Autodesk Fusion 360 part; units mm, degrees
sketch "Sketch1" plane through (0, 0, 0) normal (0, 0, 1) x (1, 0, 0)
  line L0 (60, -60) -> (-60, -60)
  line L1 (-60, -60) -> (-60, 60)
  line L2 (-60, 60) -> (60, 60)
  line L3 (60, 60) -> (60, -60)
  line L4 (60, -60) -> (-60, 60) construction
  line L5 (-60, -60) -> (60, 60) construction
  dimension "d4" = 120
  dimension "d5" = 120
extrude "Extrude1" add sketch "Sketch1" along normal blind 6
sketch "Sketch6" plane through (0, 0, 6) normal (0, 0, 1) x (-1, 0, 0)
  line L0 (-60, -60) -> (60, -60)
  line L1 (60, -60) -> (60, 60)
  line L2 (60, 60) -> (-60, 60)
  line L3 (-60, 60) -> (-60, -60)
sketch "Sketch7" plane through (0, 0, 6) normal (0, 0, 1) x (-1, 0, 0)
  line L0 (-60, -60) -> (60, -60)
  line L1 (60, -60) -> (60, 60)
  line L2 (60, 60) -> (-60, 60)
  line L3 (-60, 60) -> (-60, -60)
  line L4 (50, 60) -> (40, 60)
  line L5 (40, 60) -> (40, 70)
  line L6 (40, 70) -> (50, 70)
  line L7 (50, 70) -> (50, 60)
  circle A0 centre (45, 65) radius 1.625
  line L8 (0, -80) -> (0, 80) construction
  line L9 (75, 0) -> (-75, 0) construction
  circle A1 centre (-45, 65) radius 1.625
  line L10 (-50, 60) -> (-40, 60)
  line L11 (-40, 70) -> (-50, 70)
  line L12 (-40, 60) -> (-40, 70)
  line L13 (-50, 70) -> (-50, 60)
  line L14 (40, -70) -> (50, -70)
  line L15 (0, 80) -> (0, -80) construction
  line L16 (-40, -70) -> (-50, -70)
  line L17 (50, -60) -> (40, -60)
  circle A2 centre (-45, -65) radius 1.625
  line L18 (40, -60) -> (40, -70)
  circle A3 centre (45, -65) radius 1.625
  line L19 (50, -70) -> (50, -60)
  line L20 (-40, -60) -> (-40, -70)
  line L21 (-50, -70) -> (-50, -60)
  dimension "d78" = 10
  dimension "d79" = 10
  dimension "d80" = 10
  dimension "d81" = 3.25
  dimension "d83" = 5
  dimension "d84" = 5
extrude "Extrude7" add sketch "Sketch7" against normal up to surface (6 mm away) contours L0 L16 L20 L21 | L2 L10 L11 L12 L13 | L0 L14 L17 L18 L19 | L2 L4 L5 L6 L7
fillet "Fillet1" radius 3.5 2 edges at (-50, -70, 3) (-40, -70, 3)
fillet "Fillet2" radius 3.5 2 edges at (40, -70, 3) (50, -70, 3)
fillet "Fillet3" radius 3.5 2 edges at (-40, 70, 3) (-50, 70, 3)
fillet "Fillet4" radius 3.5 2 edges at (40, 70, 3) (50, 70, 3)
fillet "Fillet5" radius 2.5 8 edges at (50, 60, 3) (40, 60, 3) (-40, 60, 3) (-50, 60, 3) (-50, -60, 3) (50, -60, 3) (-40, -60, 3) (40, -60, 3)
fillet "Fillet6" radius 3 4 edges at (-60, 60, 3) (-60, -60, 3) (60, -60, 3) (60, 60, 3)
sketch "Sketch8" plane through (0, 0, 6) normal (0, 0, 1) x (-1, 0, 0)
  circle A0 centre (45, -65) radius 1.625
  circle A1 centre (45, 65) radius 1.625
  circle A2 centre (-45, -65) radius 1.625
  circle A3 centre (-45, 65) radius 1.625
  arc A4 (-60, -57) -> (-57, -60) centre (-57, -57) ccw
  line L0 (-57, -60) -> (-52.5, -60)
  arc A5 (-50, -62.5) -> (-52.5, -60) centre (-52.5, -62.5) ccw
  line L1 (-50, -62.5) -> (-50, -66.5)
  arc A6 (-50, -66.5) -> (-46.5, -70) centre (-46.5, -66.5) ccw
  line L2 (-46.5, -70) -> (-43.5, -70)
  arc A7 (-43.5, -70) -> (-40, -66.5) centre (-43.5, -66.5) ccw
  line L3 (-40, -66.5) -> (-40, -62.5)
  arc A8 (-37.5, -60) -> (-40, -62.5) centre (-37.5, -62.5) ccw
  line L4 (-37.5, -60) -> (37.5, -60)
  arc A9 (40, -62.5) -> (37.5, -60) centre (37.5, -62.5) ccw
  line L5 (40, -62.5) -> (40, -66.5)
  arc A10 (40, -66.5) -> (43.5, -70) centre (43.5, -66.5) ccw
  line L6 (43.5, -70) -> (46.5, -70)
  arc A11 (46.5, -70) -> (50, -66.5) centre (46.5, -66.5) ccw
  line L7 (50, -66.5) -> (50, -62.5)
  arc A12 (52.5, -60) -> (50, -62.5) centre (52.5, -62.5) ccw
  line L8 (52.5, -60) -> (57, -60)
  arc A13 (57, -60) -> (60, -57) centre (57, -57) ccw
  line L9 (60, -57) -> (60, 57)
  arc A14 (60, 57) -> (57, 60) centre (57, 57) ccw
  line L10 (57, 60) -> (52.5, 60)
  arc A15 (50, 62.5) -> (52.5, 60) centre (52.5, 62.5) ccw
  line L11 (50, 62.5) -> (50, 66.5)
  arc A16 (50, 66.5) -> (46.5, 70) centre (46.5, 66.5) ccw
  line L12 (46.5, 70) -> (43.5, 70)
  arc A17 (43.5, 70) -> (40, 66.5) centre (43.5, 66.5) ccw
  line L13 (40, 66.5) -> (40, 62.5)
  arc A18 (37.5, 60) -> (40, 62.5) centre (37.5, 62.5) ccw
  line L14 (37.5, 60) -> (-37.5, 60)
  arc A19 (-40, 62.5) -> (-37.5, 60) centre (-37.5, 62.5) ccw
  line L15 (-40, 62.5) -> (-40, 66.5)
  arc A20 (-40, 66.5) -> (-43.5, 70) centre (-43.5, 66.5) ccw
  line L16 (-43.5, 70) -> (-46.5, 70)
  arc A21 (-46.5, 70) -> (-50, 66.5) centre (-46.5, 66.5) ccw
  line L17 (-50, 66.5) -> (-50, 62.5)
  arc A22 (-52.5, 60) -> (-50, 62.5) centre (-52.5, 62.5) ccw
  line L18 (-52.5, 60) -> (-57, 60)
  arc A23 (-57, 60) -> (-60, 57) centre (-57, 57) ccw
  line L19 (-60, 57) -> (-60, -57)
  circle A24 centre (45, 65) radius 2.875
  dimension "d98" = 5.75
extrude "Extrude8" cut sketch "Sketch8" against normal blind 3.5 contours A24
sketch "Sketch9" plane through (0, 0, 6) normal (0, 0, 1) x (-1, 0, 0)
  circle A0 centre (45, 65) radius 2.875
  circle A1 centre (45, -65) radius 1.625
  circle A2 centre (-45, -65) radius 1.625
  circle A3 centre (-45, 65) radius 1.625
  arc A4 (-60, -57) -> (-57, -60) centre (-57, -57) ccw
  line L0 (-57, -60) -> (-52.5, -60)
  arc A5 (-50, -62.5) -> (-52.5, -60) centre (-52.5, -62.5) ccw
  line L1 (-50, -62.5) -> (-50, -66.5)
  arc A6 (-50, -66.5) -> (-46.5, -70) centre (-46.5, -66.5) ccw
  line L2 (-46.5, -70) -> (-43.5, -70)
  arc A7 (-43.5, -70) -> (-40, -66.5) centre (-43.5, -66.5) ccw
  line L3 (-40, -66.5) -> (-40, -62.5)
  arc A8 (-37.5, -60) -> (-40, -62.5) centre (-37.5, -62.5) ccw
  line L4 (-37.5, -60) -> (37.5, -60)
  arc A9 (40, -62.5) -> (37.5, -60) centre (37.5, -62.5) ccw
  line L5 (40, -62.5) -> (40, -66.5)
  arc A10 (40, -66.5) -> (43.5, -70) centre (43.5, -66.5) ccw
  line L6 (43.5, -70) -> (46.5, -70)
  arc A11 (46.5, -70) -> (50, -66.5) centre (46.5, -66.5) ccw
  line L7 (50, -66.5) -> (50, -62.5)
  arc A12 (52.5, -60) -> (50, -62.5) centre (52.5, -62.5) ccw
  line L8 (52.5, -60) -> (57, -60)
  arc A13 (57, -60) -> (60, -57) centre (57, -57) ccw
  line L9 (60, -57) -> (60, 57)
  arc A14 (60, 57) -> (57, 60) centre (57, 57) ccw
  line L10 (57, 60) -> (52.5, 60)
  arc A15 (50, 62.5) -> (52.5, 60) centre (52.5, 62.5) ccw
  line L11 (50, 62.5) -> (50, 66.5)
  arc A16 (50, 66.5) -> (46.5, 70) centre (46.5, 66.5) ccw
  line L12 (46.5, 70) -> (43.5, 70)
  arc A17 (43.5, 70) -> (40, 66.5) centre (43.5, 66.5) ccw
  line L13 (40, 66.5) -> (40, 62.5)
  arc A18 (37.5, 60) -> (40, 62.5) centre (37.5, 62.5) ccw
  line L14 (37.5, 60) -> (-37.5, 60)
  arc A19 (-40, 62.5) -> (-37.5, 60) centre (-37.5, 62.5) ccw
  line L15 (-40, 62.5) -> (-40, 66.5)
  arc A20 (-40, 66.5) -> (-43.5, 70) centre (-43.5, 66.5) ccw
  line L16 (-43.5, 70) -> (-46.5, 70)
  arc A21 (-46.5, 70) -> (-50, 66.5) centre (-46.5, 66.5) ccw
  line L17 (-50, 66.5) -> (-50, 62.5)
  arc A22 (-52.5, 60) -> (-50, 62.5) centre (-52.5, 62.5) ccw
  line L18 (-52.5, 60) -> (-57, 60)
  arc A23 (-57, 60) -> (-60, 57) centre (-57, 57) ccw
  line L19 (-60, 57) -> (-60, -57)
  circle A24 centre (-45, 65) radius 2.875
  circle A25 centre (-45, -65) radius 2.875
  circle A26 centre (45, -65) radius 2.875
  dimension "d101" = 5.75
  dimension "d102" = 5.75
  dimension "d103" = 5.75
extrude "Extrude9" cut sketch "Sketch9" against normal blind 3.5 contours A24 | A25 | A26
sketch "Sketch10" plane through (0, 0, 6) normal (0, 0, 1) x (-1, 0, 0)
  circle A0 centre (-45, 65) radius 2.875
  circle A1 centre (-45, -65) radius 2.875
  circle A2 centre (45, -65) radius 2.875
  circle A3 centre (45, 65) radius 2.875
  arc A4 (-60, -57) -> (-57, -60) centre (-57, -57) ccw
  line L0 (-57, -60) -> (-52.5, -60)
  arc A5 (-50, -62.5) -> (-52.5, -60) centre (-52.5, -62.5) ccw
  line L1 (-50, -62.5) -> (-50, -66.5)
  arc A6 (-50, -66.5) -> (-46.5, -70) centre (-46.5, -66.5) ccw
  line L2 (-46.5, -70) -> (-43.5, -70)
  arc A7 (-43.5, -70) -> (-40, -66.5) centre (-43.5, -66.5) ccw
  line L3 (-40, -66.5) -> (-40, -62.5)
  arc A8 (-37.5, -60) -> (-40, -62.5) centre (-37.5, -62.5) ccw
  line L4 (-37.5, -60) -> (37.5, -60)
  arc A9 (40, -62.5) -> (37.5, -60) centre (37.5, -62.5) ccw
  line L5 (40, -62.5) -> (40, -66.5)
  arc A10 (40, -66.5) -> (43.5, -70) centre (43.5, -66.5) ccw
  line L6 (43.5, -70) -> (46.5, -70)
  arc A11 (46.5, -70) -> (50, -66.5) centre (46.5, -66.5) ccw
  line L7 (50, -66.5) -> (50, -62.5)
  arc A12 (52.5, -60) -> (50, -62.5) centre (52.5, -62.5) ccw
  line L8 (52.5, -60) -> (57, -60)
  arc A13 (57, -60) -> (60, -57) centre (57, -57) ccw
  line L9 (60, -57) -> (60, 57)
  arc A14 (60, 57) -> (57, 60) centre (57, 57) ccw
  line L10 (57, 60) -> (52.5, 60)
  arc A15 (50, 62.5) -> (52.5, 60) centre (52.5, 62.5) ccw
  line L11 (50, 62.5) -> (50, 66.5)
  arc A16 (50, 66.5) -> (46.5, 70) centre (46.5, 66.5) ccw
  line L12 (46.5, 70) -> (43.5, 70)
  arc A17 (43.5, 70) -> (40, 66.5) centre (43.5, 66.5) ccw
  line L13 (40, 66.5) -> (40, 62.5)
  arc A18 (37.5, 60) -> (40, 62.5) centre (37.5, 62.5) ccw
  line L14 (37.5, 60) -> (-37.5, 60)
  arc A19 (-40, 62.5) -> (-37.5, 60) centre (-37.5, 62.5) ccw
  line L15 (-40, 62.5) -> (-40, 66.5)
  arc A20 (-40, 66.5) -> (-43.5, 70) centre (-43.5, 66.5) ccw
  line L16 (-43.5, 70) -> (-46.5, 70)
  arc A21 (-46.5, 70) -> (-50, 66.5) centre (-46.5, 66.5) ccw
  line L17 (-50, 66.5) -> (-50, 62.5)
  arc A22 (-52.5, 60) -> (-50, 62.5) centre (-52.5, 62.5) ccw
  line L18 (-52.5, 60) -> (-57, 60)
  arc A23 (-57, 60) -> (-60, 57) centre (-57, 57) ccw
  line L19 (-60, 57) -> (-60, -57)
  line L20 (-32, 32) -> (32, 32)
  line L21 (32, 32) -> (32, -32)
  line L22 (32, -32) -> (-32, -32)
  line L23 (-32, -32) -> (-32, 32)
  line L24 (-32, 32) -> (32, -32) construction
  line L25 (32, 32) -> (-32, -32) construction
  dimension "d108" = 64
  dimension "d109" = 64
extrude "Extrude10" cut sketch "Sketch10" against normal up to surface (6 mm away) contours L20 L21 L22 L23
fillet "Fillet7" radius 3 4 edges at (32, 32, 3) (32, -32, 3) (-32, 32, 3) (-32, -32, 3)
equation "base_width = 120 mm"
equation "base_length = 120 mm"
equation "base_thickness = 6 mm"
equation "d4 = base_width"
equation "d5 = base_length"
equation "d6 = base_thickness"
equation "fan_mount_hole_long_edge_offset = 18 mm"
equation "fan_bottom_mount_hole_head_countersink = 3.5 mm"
equation "fan_bottom_mount_hole_diameter = 3.25 mm"
equation "fan_bottom_mount_hole_head_diameter = 5.75 mm"
equation "fan_bottom_mount_hole_slot_length = 4 mm"
equation "fan_mount_hole_short_edge_offset = 12.5 mm"
equation "pi_mount_width = 65.7 mm"
equation "pi_mount_length = 100.7 mm"
equation "pi_bottom_mount_hole_diameter = 3.25 mm"
equation "pi_bottom_mount_hole_head_countersink = 3.5 mm"
equation "pi_bottom_mount_hole_head_diameter = 5.75 mm"
equation "pi_bottom_mount_hole_slot_length = 8 mm"
equation "switch_width = 100 mm"
equation "switch_length = 98.5 mm"
equation "switch_lateral_support_length = 10 mm"
equation "switch_lateral_support_offset = 0.4 mm"
equation "switch_lateral_support_thickness = 1 mm"
equation "switch_lateral_support_width = 2 mm"
equation "base_bracket_width = 10 mm"
equation "base_bracket_edge_offset = 10 mm"
equation "base_bracket_hole_diameter = 3.25 mm"
equation "base_bracket_length = 10 mm"
equation "base_bracket_hole_edge_offset = 5 mm"
equation "d78 = base_bracket_width"
equation "d79 = base_bracket_length"
equation "d80 = base_bracket_edge_offset"
equation "d81 = base_bracket_hole_diameter"
equation "base_bracket_length_edge_offset = 5 mm"
equation "d83 = base_bracket_length_edge_offset"
equation "d84 = base_bracket_width / 2"
equation "base_bracket_outer_fillet = 3.5 mm"
equation "base_bracket_inner_fillet = 2.5 mm"
equation "d89 = base_bracket_outer_fillet"
equation "d90 = base_bracket_outer_fillet"
equation "d91 = base_bracket_outer_fillet"
equation "d92 = base_bracket_outer_fillet"
equation "d93 = base_bracket_inner_fillet"
equation "base_edge_fillet = 3 mm"
equation "d95 = base_edge_fillet"
equation "base_bracket_bottom_mount_hole_head_countersink = 3.5 mm"
equation "base_bracket_bottom_mount_hole_head_diameter = 5.75 mm"
equation "d98 = base_bracket_bottom_mount_hole_head_diameter"
equation "d101 = base_bracket_bottom_mount_hole_head_diameter"
equation "d102 = base_bracket_bottom_mount_hole_head_diameter"
equation "d103 = base_bracket_bottom_mount_hole_head_diameter"
equation "internal_hole_width = 64 mm"
equation "internal_hole_length = 64 mm"
equation "d108 = internal_hole_width"
equation "d109 = internal_hole_length"
equation "internal_hole_fillet = 3 mm"
equation "d113 = internal_hole_fillet"
Work out the finished part from the listing and answer in its coordinate system (mm). A direction names the side the tool comes from. Coordinates: 2 decimals unless noted, no trailing zeros. Loops run counter-clockwise (first coordinate to the right, second up) from the corner with the lowest first, then second, coordinate; pieces in that order, holes last. Notation, with made-up numbers: (64.5, 60.5) -> (92.5, 60.5) arc R15 ccw to (92.5, 76.5) -> close; hole circle Ø2 at (-37, -22.75). An arc over 180 degrees is marked (long way). Write each question's results on one line, items separated by ' | '. Start each with the question number.
1) Find section D-D on z = 4.6. Count the separate pieces of the cut face and the enclosed holes in it, then the cut area to 3 significant figures.
2) The mould has two halves that part along Y. Classify faces 6 (the flat face through (-45, 70, 3)), 7 (the flat face through (-32, 0, 3)), 8 (the flat face through (55, -60, 3)): pulls with the +Y half, pulls with the -Y half, needs draft (parallel to the pull), parting line crosses it, or undercut.
3) Flat-ended cylindrical pins translate along their axes: P1, Ø3.5, axis at x = 45, y = 65, coming from the +Z side; P2, Ø3, axis at x = -28, z = 5, coming from the -Y side; P3, Ø4.5, axis at x = 46, y = -65.5, coming from the +Z side; P4, Ø3, axis at y = 64.5, z = 4, coming from the -X side. Find the tip coordinate at first contact, or state that the pin passes through.
4) For faces 1 (the flat face through (-50, 65, 3)), 2 (the flat face through (-47, -65, 2.5)), 3 (the flat face through (-60, -1, 3)), 4 (the flat face through (-40, 64, 3)), 5 (the cylindrical face through (-41, -68.95, 2.96)), determine the directions among +Z, -Z, +X, -X, +Y, -Y from which every point of the face is accessible in a straight line to the end or side of a thin tool.
5) Consider line 1 along X through (y, z) = (-65, 1.45) (3 decimals); line 2 along Y through (x, z) = (-45, 0.75) (3 decimals); line 3 along Y through (x, z) = (-45, 5) (3 decimals). Determine where each line is inside the solid, lowest interval first.
6) Find section C-C on x = 45. Determine the outline of the cut face in (y, z) (3 decimals).
7) Find section A-A on y = 3. Determine the outline of the cut face in (x, z), then the cut area to 3 significant figures.
Response values:
1) separate pieces: 1 | enclosed holes: 5 | area: 10,600 mm^2
2) face 6: pulls with the +Y half | face 7: undercut | face 8: pulls with the -Y half
3) P1: stops at z = 2.5 | P2: stops at y = -60 | P3: stops at z = 6 | P4: stops at x = -50
4) face 1: +Z, -Z, -X, +Y | face 2: +Z | face 3: +Z, -Z, -X, +Y, -Y | face 4: +Z, -Z, +Y | face 5: +Z, -Z, -Y
5) line 1: x = -50 to -46.625, -43.375 to -40, 40 to 43.375, 46.625 to 50 | line 2: y = -70 to -66.625, -63.375 to 63.375, 66.625 to 70 | line 3: y = -70 to -67.875, -62.125 to 62.125, 67.875 to 70
6) outline: (-70, 0) -> (-66.625, 0) -> (-66.625, 2.5) -> (-67.875, 2.5) -> (-67.875, 6) -> (-70, 6) -> close; (-63.375, 0) -> (63.375, 0) -> (63.375, 2.5) -> (62.125, 2.5) -> (62.125, 6) -> (-62.125, 6) -> (-62.125, 2.5) -> (-63.375, 2.5) -> close; (66.625, 0) -> (70, 0) -> (70, 6) -> (67.875, 6) -> (67.875, 2.5) -> (66.625, 2.5) -> close
7) outline: (-60, 0) -> (-32, 0) -> (-32, 6) -> (-60, 6) -> close; (32, 0) -> (60, 0) -> (60, 6) -> (32, 6) -> close | area: 336 mm^2
